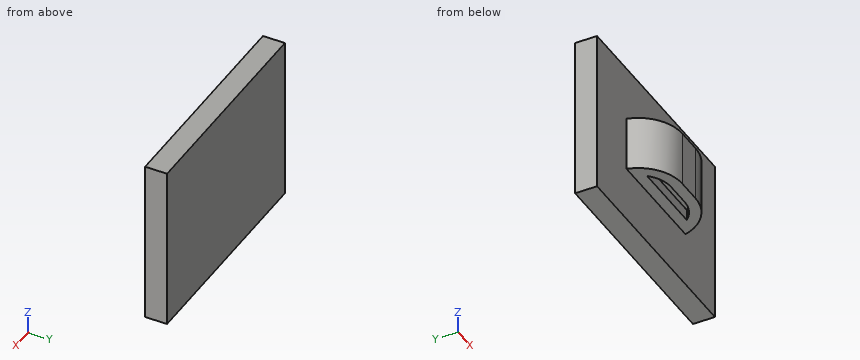
Solid Edge part; units mm, degrees
sketch "Sketch1" plane through (4.7659, 0, 3.5606) normal (0, -1, 0) x (1, 0, 0)
  line L0 (10.6791, 7.5) -> (-9.3209, 7.5)
  line L1 (-9.3209, 7.5) -> (-9.3209, -7.5)
  line L2 (-9.3209, -7.5) -> (10.6791, -7.5)
  line L3 (10.6791, -7.5) -> (10.6791, 7.5)
extrude "Protrusion1" add sketch "Sketch1" against normal blind 2
sketch "Sketch2" plane through (0, 0, 0) normal (0, -1, 0) x (1, 0, 0)
  line L0 (10.445, 6.0606) -> (0.445, 6.0606)
  line L1 (0.445, 6.0606) -> (0.445, 1.0606)
  line L2 (0.445, 1.0606) -> (10.445, 1.0606)
  line L3 (10.445, 1.0606) -> (10.445, 6.0606)
extrude "Protrusion2" add sketch "Sketch2" along normal blind 3
fillet "Round_2" radius 4 2 edges at (10.445, -3, 3.5606) (0.445, -3, 3.5606)
sketch "Sketch3" plane through (5.445, -1.5, 1.0606) normal (0, 0, -1) x (1, 0, 0)
  line L0 (-1.127, 0.5) -> (1.127, 0.5)
  arc A0 (1.127, 0.5) -> (3.3631, -0.5) centre (1.127, -2.5) cw
  line L1 (3.3631, -0.5) -> (-3.3631, -0.5)
  arc A1 (-3.3631, -0.5) -> (-1.127, 0.5) centre (-1.127, -2.5) cw
extrude "ExtrudedCutout_1" cut sketch "Sketch3" against normal blind 1
sketch "Sketch4" plane through (5.445, -1.5, 6.0606) normal (0, 0, 1) x (1, 0, 0)
  line L0 (1.127, -0.5) -> (-1.127, -0.5)
  arc A0 (-1.127, -0.5) -> (-3.3631, 0.5) centre (-1.127, 2.5) cw
  line L1 (-3.3631, 0.5) -> (3.3631, 0.5)
  arc A1 (3.3631, 0.5) -> (1.127, -0.5) centre (1.127, 2.5) cw
extrude "ExtrudedCutout_2" cut sketch "Sketch4" against normal blind 1
Build history of the part. All positions in model axes, mm. Coordinates: 2 decimals unless noted, no trailing zeros. Order: outer loops, then holes, each group sorted by start corner. A loop starts at its lowest first (then second) coordinate and runs counter-clockwise, first axis right, second up. Notation, with made-up numbers: (-4.5, 15) -> (21.5, 15) arc R9 cw to (21.5, 30) -> close; hole circle Ø10 at (49, 48). An arc over 180 degrees is marked (long way). One line per item, written item: value.
(1) Drop flat-ended pins along their axis: pin 1 Ø1.5 at (x, y) = (3.5, -0.5) entering from -Z; pin 2 Ø1.5 at (x, y) = (4.5, -1) entering from +Z; pin 3 Ø0.8 at (x, y) = (5, -1.5) entering from -Z; pin 4 Ø1.5 at (x, y) = (6.5, -1.5) entering from -Z. Give the stop position or say it passes through.
Checked values:
pin 1: z = -3.94
pin 2: z = 6.06
pin 3: z = 2.06
pin 4: z = 1.06
(2) Probe line 1 (Y direction, x = 10.75, z = 7); line 2 (Z direction, x = 8, y = -1.5); line 3 (Z direction, x = 9.5, y = -0.95). List the from-to ranges inside material, lowest first. Write a range as [from, to].
Checked values:
line 1: [0, 2]
line 2: [2.06, 5.06]
line 3: [1.06, 6.06]
(3) Slice it at D-D, the plane x = -3.25. List the corners of the cut face in (y, z).
Checked values:
outline: (0, -3.94) -> (2, -3.94) -> (2, 11.06) -> (0, 11.06) -> close
(4) Slice it at B-B, the plane z = 3. List the corners of the cut face in (x, y) (3 decimals), plus the area to 3 significant figures.
Checked values:
outline: (-4.555, 0) -> (0.445, 0) arc R4 ccw to (4.318, -3) -> (6.572, -3) arc R4 ccw to (10.445, 0) -> (15.445, 0) -> (15.445, 2) -> (-4.555, 2) -> close
area: 64.0 mm2
(5) Slice it at C-C, the plane y = -0.65. List the corners of the cut face in (x, z).
Checked values:
outline: (0.67, 1.06) -> (10.22, 1.06) -> (10.22, 6.06) -> (0.67, 6.06) -> close
(6) Slice it at A-A, the plane x = 5. List the corners of the cut face in (y, z), plus the area to 3 significant figures.
Checked values:
outline: (-3, 1.06) -> (-2, 1.06) -> (-2, 2.06) -> (-1, 2.06) -> (-1, 1.06) -> (0, 1.06) -> (0, -3.94) -> (2, -3.94) -> (2, 11.06) -> (0, 11.06) -> (0, 6.06) -> (-1, 6.06) -> (-1, 5.06) -> (-2, 5.06) -> (-2, 6.06) -> (-3, 6.06) -> close
area: 43.0 mm2
